For this review, take the finished solid that the model builds, in its own axes (mm). Face numbers are marked on the shaded views. A direction names the side the tool comes from. Give positions to 0.01 mm unless a question says otherwise; leave off trailing zeros. Order: outer loops, then holes, each group sorted by start corner. A loop starts at its lowest first (then second) coordinate and runs counter-clockwise, first axis right, second up. Notation, with made-up numbers: (54, 34) -> (75, 34) arc R29 cw to (75, 69) -> close; hole circle Ø5 at (-19, 50.5). An arc over 180 degrees is marked (long way). One line per item, written item: value. Start each with the question number.
from build123d import *

# Parameters (mm, degrees)
F1_DEPTH = 63.5
F0_W     = 25.4
F0_H     = 28.575
F2_DEPTH = 25.4
F3_DEPTH = 7.9375


# Not quite as in the source:
# - a feature of the source that left no trace in its solid (it failed there, or was rolled back) is left out


with BuildPart() as f1:
    # F0 (on Front) → F1 (new body, symmetric)
    with BuildSketch(Plane.XZ):
        Polygon((-41.275, -9.525), (41.275, -9.525), (41.275, 9.525), (22.225, 9.525), (-41.275, 9.525), align=None)
    extrude(amount=F1_DEPTH, both=True)

    # F0 (on Front) → F2 (join, symmetric)
    with BuildSketch(Plane.XZ):
        Polygon((60.325, 66.675), (60.325, 61.9252), (60.325, 42.8752), (60.325, 38.1), (85.725, 38.1), (85.725, 66.675), align=None)
        with BuildLine():
            Line((22.225, 9.525), (41.275, 9.525))
            Line((41.275, 9.525), (41.275, 27.0002))
            ThreePointArc((41.275, 27.0002), (45.9246798487, 38.2255201513), (57.15, 42.8752))
            Line((57.15, 42.8752), (60.325, 42.8752))
            Line((60.325, 42.8752), (60.325, 61.9252))
            Line((60.325, 61.9252), (57.15, 61.9252))
            ThreePointArc((57.15, 61.9252), (32.4542956671, 51.6959043329), (22.225, 27.0002))
            Line((22.225, 27.0002), (22.225, 9.525))
        make_face()
        with Locations((98.425, 52.3875)):
            Rectangle(F0_W, F0_H)
    extrude(amount=F2_DEPTH, both=True)

    # F0 (on Front) → F3 (join, symmetric)
    with BuildSketch(Plane.XZ):
        with BuildLine():
            add(Edge.make_bspline(
                [(60.325, 61.9252), (-18.8444089144, 62.9406571388), (-35.6957179924, 36.5767096935), (-41.275, 9.525)],
                knots=[0, 0, 0, 0, 114.3168446032, 114.3168446032, 114.3168446032, 114.3168446032], degree=3))
            Line((-41.275, 9.525), (22.225, 9.525))
            Line((22.225, 9.525), (22.225, 27.0002))
            ThreePointArc((22.225, 27.0002), (32.4542956671, 51.6959043329), (57.15, 61.9252))
            Line((57.15, 61.9252), (60.325, 61.9252))
        make_face()
    extrude(amount=F3_DEPTH, both=True)


solid = f1.part
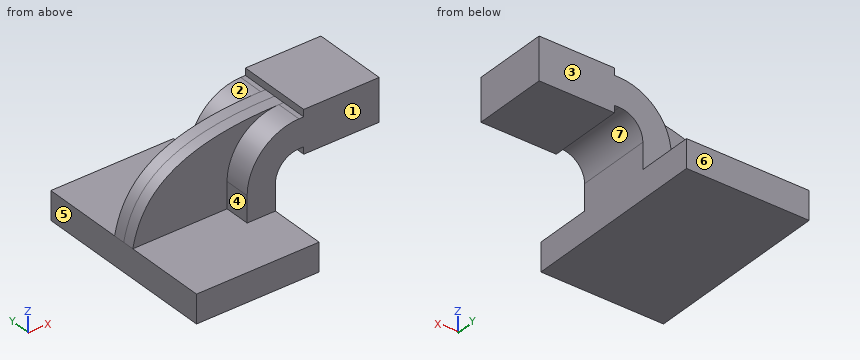
Q1. Take a section at B-B (x = 84). State the section outline as (y, z) points (3 decimals).
Q2. For line 1 along Z through (x, y) = (38, -58) (3 decimals); line 2 along Y through (x, z) = (20.5, 22.5); line 3 along Z through (x, y) = (79, -15.5) (3 decimals), list the stretches that pass through material, from the lowest coordinate up.
Q3. For the marked faces 1, 2, 3 and 4, list the 3-axis set-ups (+Z, -Z, +X, -X, +Y, -Y) from which the entire face can be reached by the end or side of a thin tool; tool diameter is ignored.
Q4. Take a section at A-A (y = -50). State the section outline as (x, z) points (3 decimals), and give its area (3 significant figures).
Q5. For pin 1 Ø10 at (y, z) = (-24.5, 43.5) entering from -X; pin 2 Ø2.5 at (x, y) = (58, -3.5) entering from -Z; pin 3 Ø2.5 at (x, y) = (59, 12.5) entering from +Z, all flat-tipped, find the tip position at first contact; note any pin that passes through.
Q6. Mouldability with a two-part tool opening along X and no side actions: class the marked faces 5, 6 and 7 as pulls with the +X half, pulls with the -X half, needs draft (parallel to the pull), parting line crosses it, or undercut.
Answers below:
1. outline: (-25.4, 38.1) -> (25.4, 38.1) -> (25.4, 66.675) -> (-25.4, 66.675) -> close
2. line 1: z = -9.525 to 9.525
2. line 2: y = -7.94 to 7.94
2. line 3: z = 38.1 to 66.675
3. face 1: +Z, +X, -X, -Y
3. face 2: +Z, -X, +Y
3. face 3: +Z, +X, -X, +Y
3. face 4: +Z, -X, -Y
4. outline: (-41.275, -9.525) -> (41.275, -9.525) -> (41.275, 9.525) -> (-41.275, 9.525) -> close
4. area: 1,570 mm²
5. pin 1: stops at x = 24.17
5. pin 2: stops at z = 42.87
5. pin 3: stops at z = 61.93
6. face 5: pulls with the -X half
6. face 6: needs draft
6. face 7: undercut
